Part model, mm, in its own coordinate system. A direction names the side the tool comes from. Give positions to 0.01 mm unless a question says otherwise; leave off trailing zeros. Order: outer loops, then holes, each group sorted by start corner. A loop starts at its lowest first (then second) coordinate and runs counter-clockwise, first axis right, second up. Notation, with made-up numbers: (-6, 44.5) -> (44, 44.5) arc R22 ccw to (44, 77.5) -> close; hole circle Ø8 at (68.5, 61.5). An arc over 180 degrees is marked (long way). Write item = value, one per line. Start each with the question number.
(1) Saw through at D-D, the plane z = -5. List the corners of the cut face in (x, y).
(2) Saw through at B-B, the plane x = 5.5. List the corners of the cut face in (y, z), then the cut area to 3 significant figures.
(3) Two-plate mould, pull along X, no slides. Class faces 4 (the flat face through (24.14, 9.86, 17.74)), 5 (the flat face through (21.55, 9.86, 12.675)), 6 (the flat face through (-2, 0, 26)): pulls with the +X half, pulls with the -X half, needs draft (parallel to the pull), parting line crosses it, or undercut.
(4) Flat gauge pins, fed straight in: pin 1 (2.5 mm diameter, centred on y = 7.5, z = -29.5, fed in from +X); pin 2 (3 mm diameter, centred on x = 0, z = 29, fed in from +Y); pin 3 (6 mm diameter, centred on y = 3, z = 8.5, fed in from +X); pin 4 (12 mm diameter, centred on x = -11, z = 7, fed in from -Y). Where does each tip first touch, or does it go through?
(5) Saw through at A-A, the plane y = 1.75. List the corners of the cut face in (x, z).
(6) Probe line 1 along Z through (x, y) = (-7.5, 14.5); line 2 along X through (y, z) = (12.5, 21); line 3 along Z through (x, y) = (-25.5, 6.75). List the from-to ranges inside material, lowest first. Write a range as from..to.
(7) Saw through at C-C, the plane y = 14.25. List the corners of the cut face in (x, z).
(8) Which spindle directions (+Z, -Z, +X, -X, +Y, -Y) get a long thin tool onto all of the face, cutting with end or side? Do faces 1 (the flat face through (0, 10, 35)), 2 (the flat face through (-21.55, 9.86, -12.675)), 3 (the flat face through (-10.25, 12, 30)). Say none if no direction does.
from build123d import *

# Parameters (mm, degrees)
SKETCH1_W           = 32.331615074
SKETCH1_H           = 7
BOSS_EXTRUDE1_DEPTH = 20
SKETCH2_W           = 20.5
SKETCH2_H           = 5.8
CUT_EXTRUDE1_DEPTH  = 17
SKETCH2_3_W         = 26
SKETCH2_3_H         = 4.8
CUT_EXTRUDE2_DEPTH  = 26


with BuildPart() as part:
    # Sketch1 → Boss-Extrude1 (new body)
    # profile 1 of 7: a face of its own
    with BuildSketch(Plane(origin=(0, 0, 0), x_dir=(1, 0, 0), z_dir=(0, 1, 0))):
        Polygon((-16.165807537, -28), (16.165807537, -28), (32.331615075, 0), (16.165807537, 28), (-16.165807537, 28), (-32.331615075, 0), align=None)
        Polygon((14.43375673, -25), (28.867513459, 0), (14.43375673, 25), (-14.43375673, 25), (-28.867513459, 0), (-14.43375673, -25), align=None, mode=Mode.SUBTRACT)
    # profile 2 of 7: a face of its own
    with BuildSketch(Plane(origin=(0, 0, 0), x_dir=(1, 0, 0), z_dir=(0, 1, 0))):
        with Locations((0, 31.5)):
            Rectangle(SKETCH1_W, SKETCH1_H)
    # profile 3 of 7: a face of its own
    with BuildSketch(Plane(origin=(0, 0, 0), x_dir=(1, 0, 0), z_dir=(0, 1, 0))):
        Polygon((-16.165807537, 28), (-32.331615075, 0), (-16.165807537, 35), align=None)
    # profile 4 of 7: a face of its own
    with BuildSketch(Plane(origin=(0, 0, 0), x_dir=(1, 0, 0), z_dir=(0, 1, 0))):
        Polygon((16.165807537, 35), (32.331615075, 0), (16.165807537, 28), align=None)
    # profile 5 of 7: a face of its own
    with BuildSketch(Plane(origin=(0, 0, 0), x_dir=(1, 0, 0), z_dir=(0, 1, 0))):
        Polygon((16.165807537, -28), (16.165807537, -35), (32.331615075, 0), align=None)
    # profile 6 of 7: a face of its own
    with BuildSketch(Plane(origin=(0, 0, 0), x_dir=(1, 0, 0), z_dir=(0, 1, 0))):
        with Locations((0, -31.5)):
            Rectangle(SKETCH1_W, SKETCH1_H)
    # profile 7 of 7: a face of its own
    with BuildSketch(Plane(origin=(0, 0, 0), x_dir=(1, 0, 0), z_dir=(0, 1, 0))):
        Polygon((-16.165807537, -35), (-32.331615075, 0), (-16.165807537, -28), align=None)
    extrude(amount=BOSS_EXTRUDE1_DEPTH)

    # Sketch2 → Cut-Extrude1 (cut)
    with BuildSketch(Plane(origin=(0, 20, 0), x_dir=(1, 0, 0), z_dir=(0, 1, 0))):
        with Locations((0, -30.3)):
            Rectangle(SKETCH2_W, SKETCH2_H)
    extrude(amount=-CUT_EXTRUDE1_DEPTH, mode=Mode.SUBTRACT)

    # Sketch2_3 → Cut-Extrude2 (cut)
    with BuildSketch(Plane(origin=(0, 20, 0), x_dir=(1, 0, 0), z_dir=(0, 1, 0))):
        with Locations((0, 30.6)):
            Rectangle(SKETCH2_3_W, SKETCH2_3_H)
    extrude(amount=-CUT_EXTRUDE2_DEPTH, mode=Mode.SUBTRACT)


solid = part.part
Results list:
q1.outline = (-30.02, 0) -> (-25.98, 0) -> (-25.98, 20) -> (-30.02, 20) -> close; (25.98, 0) -> (30.02, 0) -> (30.02, 20) -> (25.98, 20) -> close
q2.outline = (0, -35) -> (20, -35) -> (20, -33) -> (0, -33) -> close; (0, -28.2) -> (20, -28.2) -> (20, -25) -> (0, -25) -> close; (0, 25) -> (20, 25) -> (20, 27.4) -> (3, 27.4) -> (3, 33.2) -> (20, 33.2) -> (20, 35) -> (0, 35) -> close
q2.area = 205 mm^2
q3.face_4 = pulls with the +X half
q3.face_5 = undercut
q3.face_6 = needs draft
q4.pin_1 = 19.28
q4.pin_2 = 3
q4.pin_3 = 29.79
q4.pin_4 = through
q5.outline = (-32.33, 0) -> (-16.17, -35) -> (16.17, -35) -> (32.33, 0) -> (16.17, 35) -> (-16.17, 35) -> close; hole (-28.87, 0) -> (-14.43, -25) -> (14.43, -25) -> (28.87, 0) -> (14.43, 25) -> (-14.43, 25) -> close; hole (-13, -33) -> (13, -33) -> (13, -28.2) -> (-13, -28.2) -> close
q6.line_1 = -35..-33, -28.2..-25, 25..27.4, 33.2..35
q6.line_2 = -22.63..-16.74, 16.74..22.63
q6.line_3 = -14.79..-5.83, 5.83..14.79
q7.outline = (-32.33, 0) -> (-16.17, -35) -> (16.17, -35) -> (32.33, 0) -> (16.17, 35) -> (-16.17, 35) -> close; hole (-28.87, 0) -> (-14.43, -25) -> (14.43, -25) -> (28.87, 0) -> (14.43, 25) -> (-14.43, 25) -> close; hole (-13, -33) -> (13, -33) -> (13, -28.2) -> (-13, -28.2) -> close; hole (-10.25, 27.4) -> (10.25, 27.4) -> (10.25, 33.2) -> (-10.25, 33.2) -> close
q8.face_1 = +Z, +X, -X, +Y, -Y
q8.face_2 = +Y, -Y
q8.face_3 = +Y
